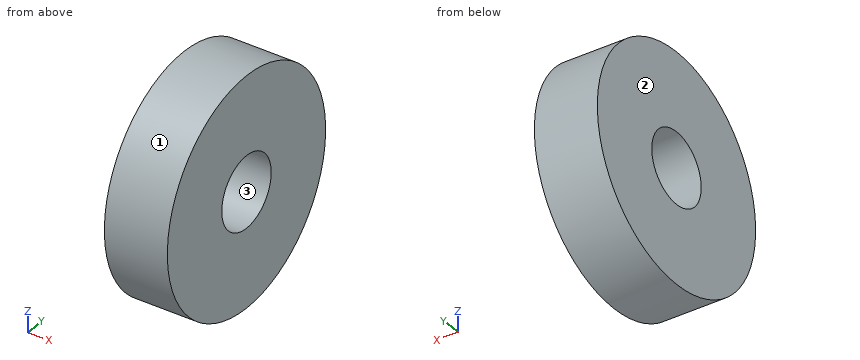
from build123d import *

# Parameters (mm, degrees)
SKETCH001_R         = 3.96875
EXTRUDE001_DEPTH    = 7
SKETCH_R            = 12.7
EXTRUDE_DEPTH       = 7
CUT_PLACEMENT_ANGLE = 90


with BuildPart() as extrude001:
    # Sketch001 (on Face2 of Extrude) → Extrude001 (new body)
    with BuildSketch(Plane(origin=(0, 0, 0), x_dir=(1, 0, 0), z_dir=(0, 0, -1))):
        Circle(SKETCH001_R)
    extrude(amount=-EXTRUDE001_DEPTH)


with BuildPart() as obj1:
    # Sketch → Extrude (new body)
    with BuildSketch(Plane.XY):
        Circle(SKETCH_R)
    extrude(amount=EXTRUDE_DEPTH)

    # Cut: cut Extrude001
    add(extrude001.part, mode=Mode.SUBTRACT)


with BuildPart() as obj1_1:
    # Cut placement: moved
    add(obj1.part.rotate(Axis((0, 0, 0), (0, 1, 0)), CUT_PLACEMENT_ANGLE))


solid = obj1_1.part
Design review of the part built by this model. Coordinates are the model's own, in mm. Face numbers are marked on the shaded views. Give positions to 0.01 mm unless a question says otherwise; leave off trailing zeros. Write each loop counter-clockwise with the first axis right and the second up, starting at its lowest first coordinate (ties: lowest second). Pieces come first, ordered by that corner, then holes. Notation, with made-up numbers: M -10,-24 L -3,-24 A22 cw -3,0 Z; hole C -4.75,36.5 d5. An arc over 180 degrees is marked long. Answer as a JSON object with one key per item and string values. Group by question number.
1) Clearance check with flat-ended pins moving along their axes: pin 1 Ø1 at (x, y) = (4, 2.5) entering from -Z; pin 2 Ø4 at (x, y) = (2.5, 6) entering from +Z; pin 3 Ø3 at (x, z) = (5, -5) entering from +Y. State where each tip first meets the part, or that it passes through.
2) We need section D-D (z = -6). Give the boundary of the cut face in (x, y).
3) We need section C-C (x = 4.75). Give the boundary of the cut face in (y, z).
4) For line 1 along Y through (x, z) = (3.5, 0); line 2 along Z through (x, y) = (3.25, 2.25), list the stretches that pass through material, from the lowest coordinate up.
5) We need section A-A (z = 0). Give the boundary of the cut face in (x, y).
6) Mouldability with a two-part tool opening along Z and no side actions: class the marked faces 1, 2 and 3 as released by +Z, released by -Z, zero draft, split by the parting line, or undercut.
Answer key:
{
 "1": {"pin 1": "stops at z = -12.54", "pin 2": "stops at z = 12.05", "pin 3": "stops at y = 12.21"},
 "2": {"outline": "M 0,-11.19 L 7,-11.19 L 7,11.19 L 0,11.19 Z"},
 "3": {"outline": "C 0,0 d25.4; hole C 0,0 d7.94"},
 "4": {"line 1": "y = -12.7 to -3.97, 3.97 to 12.7", "line 2": "z = -12.5 to -3.27, 3.27 to 12.5"},
 "5": {"outline": "M 0,-12.7 L 7,-12.7 L 7,-3.97 L 0,-3.97 Z; M 0,3.97 L 7,3.97 L 7,12.7 L 0,12.7 Z"},
 "6": {"face 1": "split by the parting line", "face 2": "zero draft", "face 3": "undercut"}
}
